```python
from build123d import *


with BuildPart() as part:
    # Sketch1 → Revolve1 (revolve)
    with BuildSketch(Plane.XY, mode=Mode.PRIVATE) as revolve1_sk:
        Polygon((-125, 0), (-125, 3.75), (-115, 3.75), (-115, 7.5), (-100, 7.5), (-100, 20), (-98.5, 20), (-98.5, 7.5), (-38, 7.5), (-38, 20), (-36.5, 20), (-36.5, 7.5), (-6.5, 7.5), (-6.5, 22), (-5, 22), (-5, 21), (5, 21), (5, 22), (6.5, 22), (6.5, 7.5), (36.5, 7.5), (36.5, 20), (38, 20), (38, 7.5), (98.5, 7.5), (98.5, 20), (100, 20), (100, 7.5), (115, 7.5), (115, 3.75), (125, 3.75), (125, 0), align=None)
    revolve(revolve1_sk.sketch.rotate(Axis((-7.951807229, 0, 0), (-1, 0, 0)), 90), axis=Axis((-7.951807229, 0, 0), (-1, 0, 0)))


solid = part.part
```
Check sheet for the modelled part. Datum: model origin and axes. Units: mm. A direction names the side the tool comes from. Coordinates: 2 decimals unless noted, no trailing zeros. Loops run counter-clockwise (first coordinate to the right, second up) from the corner with the lowest first, then second, coordinate; pieces in that order, holes last.
1) Release check for a two-part mould opening along X. For faces 4 (the face through (-5.74, 21.477, 4.769)), 5 (the face through (98.5, 0, 9)), 6 (the face through (115, 3, -3)) record: released by +X, released by -X, zero draft, split by the parting line, or undercut.
2) Gauge pin test, flat ends, axial feed: pin 1 (1.5 mm diameter, centred on x = 33.5, z = 5, fed in from +Y); pin 2 (13 mm diameter, centred on y = -10.5, z = 10, fed in from -X); pin 3 (3 mm diameter, centred on x = -38, z = -2, fed in from -Y). Record the tip position at first contact, or that the pin passes through.
3) Sectioned sample at A-A (y = 17). Record the boundary of the cut face in (x, z).
4) Access from +Z, -Z, +X, -X, +Y, -Y to the whole of each face (thin tool, end or side, straight path). Record for faces 1 (the face through (100, 0, -9)), 2 (the face through (-37.24, -0.88, 19.98)), 3 (the face through (6.5, 9, 0)).
5) Material ranges on probe 1 along X at (y, z) = (-7, -16.5); probe 2 along X at (y, z) = (14, -16.5); probe 3 along X at (y, z) = (20, 3.5), recorded low to high.
6) Sectioned sample at C-C (x = -84). Record the boundary of the cut face in (y, z).
Check sheet entries:
1. face 4: zero draft
1. face 5: undercut
1. face 6: released by +X
2. pin 1: stops at y = 6.18
2. pin 2: stops at x = -100
2. pin 3: stops at y = -19.99
3. outline: (-100, -10.54) - (-98.5, -10.54) - (-98.5, 10.54) - (-100, 10.54) - close; (-38, -10.54) - (-36.5, -10.54) - (-36.5, 10.54) - (-38, 10.54) - close; (-6.5, -13.96) - (-5, -13.96) - (-5, -12.33) - (5, -12.33) - (5, -13.96) - (6.5, -13.96) - (6.5, 13.96) - (5, 13.96) - (5, 12.33) - (-5, 12.33) - (-5, 13.96) - (-6.5, 13.96) - close; (36.5, -10.54) - (38, -10.54) - (38, 10.54) - (36.5, 10.54) - close; (98.5, -10.54) - (100, -10.54) - (100, 10.54) - (98.5, 10.54) - close
4. face 1: +X
4. face 2: -X
4. face 3: none
5. probe 1: x = -100 to -98.5, -38 to -36.5, -6.5 to 6.5, 36.5 to 38, 98.5 to 100
5. probe 2: x = -6.5 to -5, 5 to 6.5
5. probe 3: x = -6.5 to 6.5
6. outline: circle Ø15 at (0, 0)
